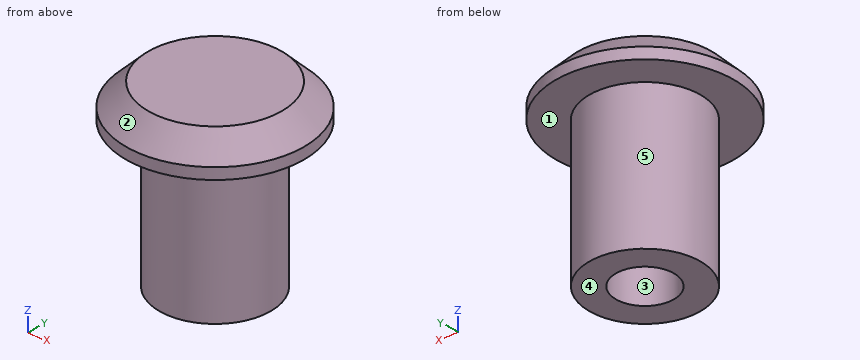
Autodesk Inventor part; units mm, degrees
ref_plane "YZ Plane" through (0, 0, 0) normal (1, 0, 0) x (0, 1, 0)
ref_plane "XZ Plane" through (0, 0, 0) normal (0, 1, 0) x (-1, 0, 0)
ref_plane "XY Plane" through (0, 0, 0) normal (0, 0, 1) x (1, 0, 0)
sketch "Sketch1" plane through (0, 0, 0) normal (0, 0, 1) x (1, 0, 0)
  circle A0 centre (0, 0) radius 1.3
  circle A1 centre (0, 0) radius 2.49
  dimension "d0" = 2.6
  dimension "d1" = 4.98
extrude "Extrusion1" add sketch "Sketch1" along normal blind 6.5 contours A0 | A1
sketch "Sketch2" plane through (0, 0, 6.5) normal (0, 0, 1) x (1, 0, 0)
  circle A0 centre (0, 0) radius 2.49
  circle A1 centre (0, 0) radius 3.99
  circle A2 centre (0, 0) radius 2.49
  dimension "d4" = 1.5
extrude "Extrusion2" add sketch "Sketch2" along normal blind 1.5 contours A0 | A1
extrude "Extrusion3" cut sketch "Sketch1" along normal blind 6 contours A0
chamfer "Chamfer1" distance 1 angle 45 1 edges at (-3.99, 0, 8)
properties part number "steering_bolt"
Here's how the part is built. I have some questions about the finished solid (model axes, mm). Face numbers are marked on the shaded views. A direction names the side the tool comes from. Round coordinates to 2 decimals unless told otherwise and drop trailing zeros. Order: outer loops, then holes, each group sorted by start corner. A loop starts at its lowest first (then second) coordinate and runs counter-clockwise, first axis right, second up. Notation, with made-up numbers: M 70,-7.75 L 101,-7.75 A20 ccw 101,-2.75 Z; hole C 7,21.5 d6. An arc over 180 degrees is marked long. Return JSON: item names as keys, results as strings. Group by question number.
1. On a 3-axis mill with a long thin cutter (end or side, diameter ignored), from which of +Z, -Z, +X, -X, +Y, -Y can I reach the whole of each face in a straight line? I mean the marked faces 4 and 5. Say none if no direction works.
2. If we section it at A-A on x = 0: List the corners of the cut face in (y, z) for me.
3. Please list where these lines run through material, in increasing order: probe 1 along Y at (x, z) = (0, 1.6); probe 2 along Z at (x, y) = (2.5, -1); probe 3 along Y at (x, z) = (0.5, 1).
4. If we section it at C-C on z = 0.5: List the corners of the cut face in (x, y) for me, then the cut area to 3 significant figures.
5. If we mould it in two halves opening along Y, with no side actions, what happens to the marked faces 1, 2 and 3? For each: pulls with the +Y half, pulls with the -Y half, needs draft (parallel to the pull), parting line crosses it, or undercut.
6. I'm going to push flat-ended pins straight in: pin 1 Ø1.5 at (x, y) = (-3, 3) entering from -Z; pin 2 Ø1.3 at (x, y) = (0, -0.5) entering from -Z; pin 3 Ø3 at (y, z) = (0, 1.5) entering from -X. Where does each tip first touch, or does it pass through?
Reply:
{
 "1": {"face 4": "-Z, +X, -X, +Y, -Y", "face 5": "-Z"},
 "2": {"outline": "M -3.99,6.5 L -2.49,6.5 L -2.49,0 L -1.3,0 L -1.3,6 L 1.3,6 L 1.3,0 L 2.49,0 L 2.49,6.5 L 3.99,6.5 L 3.99,7 L 2.99,8 L -2.99,8 L -3.99,7 Z"},
 "3": {"probe 1": "-2.49 to -1.3, 1.3 to 2.49", "probe 2": "6.5 to 8", "probe 3": "-2.44 to -1.2, 1.2 to 2.44"},
 "4": {"outline": "C 0,0 d4.98; hole C 0,0 d2.6", "area": "14.2 mm^2"},
 "5": {"face 1": "needs draft", "face 2": "parting line crosses it", "face 3": "undercut"},
 "6": {"pin 1": "z = 6.5", "pin 2": "z = 6", "pin 3": "x = -2.49"}
}
